```python
from build123d import *

# Parameters (mm, degrees)
SKETCH_1_R          = 10
EXTRUDE_1_DEPTH     = 20
CUT_EXTRUDE_1_DEPTH = 12
SKETCH_3_R          = 10
EXTRUDE_2_DEPTH     = 27


with BuildPart() as part:
    # 草图1 → 凸台-拉伸1 (new, symmetric)
    with BuildSketch(Plane.XY):
        with BuildLine():
            Line((40, 55), (18.91891904, -6.48648649))
            ThreePointArc((18.91891904, -6.48648649), (-3.287979748, -19.727878593), (-20.000000115, 0))
            Line((-20.000000115, 0), (-20.000000115, 55))
            Line((-20.000000115, 55), (-20.000000115, 63))
            Line((-20.000000115, 63), (40, 63))
            Line((40, 63), (40, 55))
        make_face()
        Circle(SKETCH_1_R, mode=Mode.SUBTRACT)
    extrude(amount=EXTRUDE_1_DEPTH, both=True)

    # 草图2 → 切除-拉伸1 (cut, symmetric)
    with BuildSketch(Plane.XY):
        with BuildLine():
            Line((18.91891904, -6.48648649), (40, 55))
            Line((40, 55), (-20.000000115, 55))
            Line((-20.000000115, 55), (-20.000000115, 0))
            ThreePointArc((-20.000000115, 0), (-3.287979748, -19.727878593), (18.91891904, -6.48648649))
        make_face()
    extrude(amount=CUT_EXTRUDE_1_DEPTH, both=True, mode=Mode.SUBTRACT)

    # 草图3 → 凸台-拉伸2 (add)
    with BuildSketch(Plane(origin=(0, 63, 0), x_dir=(1, 0, 0), z_dir=(0, 1, 0))):
        with Locations(Location((0, 0, 0), (0, 0, 90))):
            Circle(SKETCH_3_R)
    extrude(amount=EXTRUDE_2_DEPTH)


solid = part.part
```
Verification items for the finished model (mm, model axes). A direction names the side the tool comes from. Round coordinates to 2 decimals unless told otherwise and drop trailing zeros. Loops run counter-clockwise (first coordinate to the right, second up) from the corner with the lowest first, then second, coordinate; pieces in that order, holes last. Notation, with made-up numbers: (28, -39.75) -> (58, -39.75) arc R13 ccw to (58, -17.75) -> close; hole circle Ø2 at (28.5, -13). An arc over 180 degrees is marked (long way). Answer as a JSON object with one key per item and string values.
Q1. Go/stop test with flat-tipped pins: P1, Ø1.5, axis at x = 4.5, z = -15, coming from the +Y side; P2, Ø19, axis at x = 13.5, z = 3, coming from the -Y side. Record where each tip stops, or that it passes through.
Data:
{"P1": "stops at y = 63", "P2": "stops at y = -17.05"}
Q2. Section check C-C (z = 0). Record the boundary of the cut face in (x, y), then the cut area to 3 significant figures.
Data:
{"outline": "(-20, 55) -> (40, 55) -> (40, 63) -> (10, 63) -> (10, 90) -> (-10, 90) -> (-10, 63) -> (-20, 63) -> close", "area": "1,020 mm2"}
Q3. Section check A-A (x = 0). Record the boundary of the cut face in (y, z).
Data:
{"outline": "(-20, -20) -> (-10, -20) -> (-10, -12) -> (-20, -12) -> close; (-20, 12) -> (-10, 12) -> (-10, 20) -> (-20, 20) -> close; (10, -20) -> (63, -20) -> (63, -10) -> (90, -10) -> (90, 10) -> (63, 10) -> (63, 20) -> (10, 20) -> (10, 12) -> (55, 12) -> (55, -12) -> (10, -12) -> close"}
Q4. Draft check along Z on faces 3 (the flat face through (3, 26, 12)), 4 (the cylindrical face through (-2.17, -9.76, 15.94)), 5 (the cylindrical face through (9.76, 76.31, 2.17)). Enter one of: pulls with the +Z half, pulls with the -Z half, needs draft (parallel to the pull), parting line crosses it, or undercut.
Data:
{"face 3": "undercut", "face 4": "needs draft", "face 5": "parting line crosses it"}
Q5. Section check B-B (y = 31.5). Record the boundary of the cut face in (x, z).
Data:
{"outline": "(-20, -20) -> (31.94, -20) -> (31.94, -12) -> (-20, -12) -> close; (-20, 12) -> (31.94, 12) -> (31.94, 20) -> (-20, 20) -> close"}
Q6. Access from +Z, -Z, +X, -X, +Y, -Y to the whole of each face (thin tool, end or side, straight path). Record for faces 1 (the flat face through (3, 26, -12)), 2 (the flat face through (29.61, 24.69, 16.06)).
Data:
{"face 1": "+X, -X, -Y", "face 2": "+Z, -Z, +X, -Y"}
Q7. Section check D-D (x = -14.5). Record the boundary of the cut face in (y, z).
Data:
{"outline": "(-13.77, -20) -> (63, -20) -> (63, 20) -> (-13.77, 20) -> (-13.77, 12) -> (55, 12) -> (55, -12) -> (-13.77, -12) -> close"}
Q8. Scan lines: line 1 (Z direction, x = -5.5, y = -8.5); line 2 (Y direction, x = 0, z = -16.25); line 3 (Y direction, x = -7, z = 3.5). Record each from-to range of solid material in increasing order. Write a range as from..to.
Data:
{"line 1": "z = -20..-12, 12..20", "line 2": "y = -20..-10, 10..63", "line 3": "y = 55..90"}
